CAD build for the part. Positions are in the model's coordinates, mm. A direction names the side the tool comes from. Round coordinates to 2 decimals unless told otherwise and drop trailing zeros. Order: outer loops, then holes, each group sorted by start corner. A loop starts at its lowest first (then second) coordinate and runs counter-clockwise, first axis right, second up. Notation, with made-up numbers: M -13,-12 L 19,-12 A28 cw 19,16 Z; hole C 76.5,84 d10. An arc over 180 degrees is marked long. Answer as a JSON object with one key per item and string values.
```python
from build123d import *

# Parameters (mm, degrees)
SKETCH_1_R      = 1
EXTRUDE_1_DEPTH = 0.5
EXTRUDE1_START  = -0.5
EXTRUDE1_DEPTH  = 1
EXTRUDE2_DEPTH  = 0.5
FILLET2_R       = 1.6
FILLET3_R       = 3.2


# Read off the part's stored shape, not the designer's step: Extrude1
with BuildPart() as part:
    # Sketch 1 → Extrude 1 (new, symmetric)
    with BuildSketch(Plane.XY):
        with BuildLine():
            Line((0, 2), (-25.5979, 2))
            ThreePointArc((-25.5979, 2), (-27.5979, 0), (-25.5979, -2))
            Line((-25.5979, -2), (0, -2))
            ThreePointArc((0, -2), (2, 0), (0, 2))
        make_face()
        with Locations((-25.5979, 0)):
            Circle(SKETCH_1_R, mode=Mode.SUBTRACT)
        Circle(SKETCH_1_R, mode=Mode.SUBTRACT)
    extrude(amount=EXTRUDE_1_DEPTH, both=True)

    # Extrude1 outline → Extrude1 (add)
    with BuildSketch(Plane.XY.offset(EXTRUDE1_START)):
        with BuildLine():
            ThreePointArc((-9.154212394, 2), (-13.9, 5.15), (-18.645787606, 2))
            Line((-18.645787606, 2), (-9.154212394, 2))
        make_face()
    extrude(amount=EXTRUDE1_DEPTH)

    # Sketch → Extrude2 (cut, symmetric)
    with BuildSketch(Plane.XY):
        with BuildLine():
            Line((-16.113594362, 4.65), (-13.9, 4.65))
            Line((-13.9, 4.65), (-13.9, 5.15))
            ThreePointArc((-13.9, 5.15), (-15.034680572, 5.023445033), (-16.113594362, 4.65))
        make_face()
        with BuildLine():
            Line((-13.9, 4.65), (-11.686405638, 4.65))
            ThreePointArc((-11.686405638, 4.65), (-12.765319428, 5.023445033), (-13.9, 5.15))
            Line((-13.9, 5.15), (-13.9, 4.65))
        make_face()
        with BuildLine():
            Line((-13.9, 0), (-11.75, 0))
            ThreePointArc((-11.75, 0), (-11.782663331, 0.373343582), (-11.879660865, 0.735343308))
            ThreePointArc((-11.879660865, 0.735343308), (-12.140166364, 1.235105491), (-12.521595125, 1.65))
            Line((-12.521595125, 1.65), (-13.9, 1.65))
            Line((-13.9, 1.65), (-15.278404875, 1.65))
            ThreePointArc((-15.278404875, 1.65), (-15.659833636, 1.235105491), (-15.920339135, 0.735343308))
            ThreePointArc((-15.920339135, 0.735343308), (-15.860511069, -0.882551045), (-14.688986692, -2))
            Line((-14.688986692, -2), (-13.9, -2))
            Line((-13.9, -2), (-13.9, 0))
        make_face()
        with BuildLine():
            Line((-16.915922679, -2), (-14.688986692, -2))
            ThreePointArc((-14.688986692, -2), (-15.860511069, -0.882551045), (-15.920339135, 0.735343308))
            Line((-15.920339135, 0.735343308), (-16.915922679, -2))
        make_face()
        with BuildLine():
            Line((-11.612017789, 0), (-11.75, 0))
            ThreePointArc((-11.75, 0), (-12.12252688, -1.209582286), (-13.111013308, -2))
            Line((-13.111013308, -2), (-10.884077321, -2))
            Line((-10.884077321, -2), (-11.612017789, 0))
        make_face()
        with BuildLine():
            ThreePointArc((-13.111013308, -2), (-12.12252688, -1.209582286), (-11.75, 0))
            Line((-11.75, 0), (-13.9, 0))
            Line((-13.9, 0), (-13.9, -2))
            Line((-13.9, -2), (-13.111013308, -2))
        make_face()
        with BuildLine():
            ThreePointArc((-11.879660865, 0.735343308), (-11.782663331, 0.373343582), (-11.75, 0))
            Line((-11.75, 0), (-11.612017789, 0))
            Line((-11.612017789, 0), (-11.879660865, 0.735343308))
        make_face()
    extrude(amount=EXTRUDE2_DEPTH, both=True, mode=Mode.SUBTRACT)

    # Fillet2
    fillet2_edges = [part.edges().sort_by_distance(p)[0] for p in [
        (-18.645787606, 2, 0),
        (-9.154212394, 2, 0),
        (-15.278404875, 1.65, 0),
        (-12.521595125, 1.65, 0),
    ]]
    fillet(fillet2_edges, radius=FILLET2_R)

    # Fillet3
    fillet3_edges = [part.edges().sort_by_distance(p)[0] for p in [
        (-11.686405638, 4.65, 0),
        (-16.113594362, 4.65, 0),
        (-10.884077321, -2, 0),
        (-16.915922679, -2, 0),
    ]]
    fillet(fillet3_edges, radius=FILLET3_R)


solid = part.part
```
Item 1: Saw through at B-B on x = -5.75. List the corners of the cut face in (y, z).
Worked answers:
{"outline": "M -2,-0.5 L 2,-0.5 L 2,0.5 L -2,0.5 Z"}
Item 2: Saw through at A-A on z = -0.2. State how many separate pieces and enclosed holes the cut face has, and give its area (3 significant figures).
Worked answers:
{"separate pieces": "1", "enclosed holes": "2", "area": "110 mm2"}
Item 3: Two-plate mould, pull along X, no slides. Class faces 5 (the cylindrical face through (-18.827, 2.205, 0.007)), 6 (the flat face through (-14, 4.65, 0)), 7 (the cylindrical face through (0, -1, 0)): released by +X, released by -X, zero draft, split by the parting line, or undercut.
Worked answers:
{"face 5": "released by -X", "face 6": "zero draft", "face 7": "undercut"}
Item 4: Wall check: line 1 along X through (y, z) = (1.5, 0.2); line 2 along Y through (x, z) = (-3.75, 0.05); line 3 along X through (y, z) = (4, 0.25). Give the ranges that are in metal, low to high. Write a range as [from, to].
Worked answers:
{"line 1": "x = [-26.92, -15.14], [-12.66, 1.32]", "line 2": "y = [-2, 2]", "line 3": "x = [-17.14, -10.66]"}
Item 5: 3-axis set-ups, long thin cutter, end or side, ignore diameter. For faces 1 (the cylindrical face through (-24.674, -0.383, -0.007)), 2 (the flat face through (-23, 2, 0)), 3 (the flat face through (-4, 2, 0)), 4 (the flat face through (-14, 1.65, 0)): which of +Z, -Z, +X, -X, +Y, -Y reach the whole face in a straight line?
Worked answers:
{"face 1": "+Z, -Z", "face 2": "+Z, -Z, -X, +Y", "face 3": "+Z, -Z, +X, +Y", "face 4": "+Z, -Z, -Y"}
